Read the model definition and answer for the solid it produces. Units are mm, in the model's axes. A direction names the side the tool comes from. Coordinates: 2 decimals unless noted, no trailing zeros. Loops run counter-clockwise (first coordinate to the right, second up) from the corner with the lowest first, then second, coordinate; pieces in that order, holes last. Notation, with made-up numbers: M 28.25,6.25 L 81.25,6.25 A5 cw 81.25,14.25 Z; hole C 52,68 d10. An arc over 180 degrees is marked long. One line per item, written item: value. Start each with the question number.
1. Consider probe 1 along Z at (x, y) = (0, 6.75); probe 2 along Z at (x, y) = (0, 8.4). Determine where each line is inside the solid, lowest interval first.
2. The part is cut by section C-C (y = 9.5). Write down the section's boundary in (x, z).
3. Determine the mould class of faces 1 (the face through (-1.5, 3.97, 0.07)), 2 (the face through (2.87, 3.97, -2.64)), 3 (the face through (3, 8.05, 3)) for opening direction X: +X half, -X half, draft (parallel to the pull), parting line (faces both ways), or undercut.
4. For faces 4 (the face through (-2, 0, 0)), 5 (the face through (2, 8.05, 0)), determine the directions among +Z, -Z, +X, -X, +Y, -Y from which every point of the face is accessible in a straight line to the end or side of a thin tool.
5. The part is cut by section B-B (x = 0). Write down the section's boundary in (y, z).
6. Flat-ended cylindrical pins translate along their axes: pin 1 (2 mm diameter, centred on x = -0.5, y = 8.5, fed in from +Z); pin 2 (2.5 mm diameter, centred on x = 1, z = -1, fed in from +Y); pin 3 (4.5 mm diameter, centred on x = 0, z = 0, fed in from +Y); pin 4 (6 mm diameter, centred on y = 7.5, z = 5.5, fed in from -X). Find the tip coordinate at first contact, or state that the pin passes through.
7. The part is cut by section A-A (z = 0). Write down the section's boundary in (x, y), then the cut area to 3 significant figures.
8. The part is cut by section D-D (z = -6.25). Write down the section's boundary in (x, y), then the cut area to 3 significant figures.
Autodesk Inventor part; units mm, degrees
ref_plane "YZ Plane" through (0, 0, 0) normal (1, 0, 0) x (0, 1, 0)
ref_plane "XZ Plane" through (0, 0, 0) normal (0, 1, 0) x (-1, 0, 0)
ref_plane "XY Plane" through (0, 0, 0) normal (0, 0, 1) x (1, 0, 0)
sketch "Эскиз1" plane through (0, 0, 0) normal (0, 1, 0) x (-1, 0, 0)
  circle A0 centre (0, 0) radius 3.9
  dimension "d0" = 7.8
extrude "Выдавливание1" add sketch "Эскиз1" along normal blind 8.05
sketch "Эскиз2" plane through (0, 8.05, 0) normal (0, 1, 0) x (1, 0, 0)
  circle A0 centre (0, 0) radius 1.5
  dimension "d3" = 3
extrude "Выдавливание2" cut sketch "Эскиз2" against normal blind 8.05
sketch "Эскиз3" plane through (0, 8.05, 0) normal (0, 1, 0) x (1, 0, 0)
  circle A0 centre (0, 0) radius 14
  circle A1 centre (0, 0) radius 1.5
  dimension "d6" = 28
extrude "Выдавливание3" add sketch "Эскиз3" along normal blind 3
sketch "Эскиз4" plane through (0, 11.05, 0) normal (0, 1, 0) x (1, 0, 0)
  circle A0 centre (0, 0) radius 2.5
  dimension "d9" = 5
extrude "Выдавливание4" cut sketch "Эскиз4" against normal blind 3
chamfer "Фаска1" distance 2 angle 45 1 edges at (-2.5, 11.05, 0)
properties part number "000.005.002.003 - ВТУЛКА" material "Пластик АБС"
Answer block:
1. probe 1: z = -3.9 to -1.5, 1.5 to 3.9
1. probe 2: z = -14 to -2.5, 2.5 to 14
2. outline: C 0,0 d28; hole C 0,0 d5.9
3. face 1: undercut
3. face 2: parting line
3. face 3: draft
4. face 4: +Z, -Z, +X, -X, -Y
4. face 5: +Y
5. outline: M 0,-3.9 L 8.05,-3.9 L 8.05,-14 L 11.05,-14 L 11.05,-4.5 L 9.05,-2.5 L 8.05,-2.5 L 8.05,-1.5 L 0,-1.5 Z; M 0,1.5 L 8.05,1.5 L 8.05,2.5 L 9.05,2.5 L 11.05,4.5 L 11.05,14 L 8.05,14 L 8.05,3.9 L 0,3.9 Z
6. pin 1: stops at z = 14
6. pin 2: stops at y = 9.21
6. pin 3: stops at y = 8.05
6. pin 4: stops at x = -13.77
7. outline: M -14,8.05 L -3.9,8.05 L -3.9,0 L -1.5,0 L -1.5,8.05 L -2.5,8.05 L -2.5,9.05 L -4.5,11.05 L -14,11.05 Z; M 1.5,0 L 3.9,0 L 3.9,8.05 L 14,8.05 L 14,11.05 L 4.5,11.05 L 2.5,9.05 L 2.5,8.05 L 1.5,8.05 Z
7. area: 104 mm2
8. outline: M -12.53,8.05 L 12.53,8.05 L 12.53,11.05 L -12.53,11.05 Z
8. area: 75.2 mm2
